Input: dimensioned drawing with shaded views. Units: mm. Origin: part minimum x, y, z. Give positions to 0.01 mm unless a question says otherwise; leave off trailing zeros. Order: outer loops, then holes, each group sorted by start corner. A loop starts at its lowest first (then second) coordinate and runs counter-clockwise, first axis right, second up. Notation, with made-up numbers: M -10.5,31.25 L 46.5,31.25 A15 cw 46.5,45.25 Z; hole C -3,82.25 d10. An arc over 180 degrees is marked long. Answer in a Markdown table with one row per item. Add a question column.
(1) Section query A-A, the plane y = 5. Return loops of the section in (x, z), plus the area to 3 significant figures.
(2) Section query C-C, the plane x = 18. Return loops of the section in (y, z), plus the area to 3 significant figures.
(3) Pin query (flat end, axial travel): P1, Ø2.5, axis at y = 5, z = 5, coming from the -X side. Return the tip coordinate at first contact, or that it passes through.
(4) Material intervals for line 1 along Y through (x, z) = (22.5, 5); line 2 along Y through (x, z) = (74.5, 6), sorted ascending.
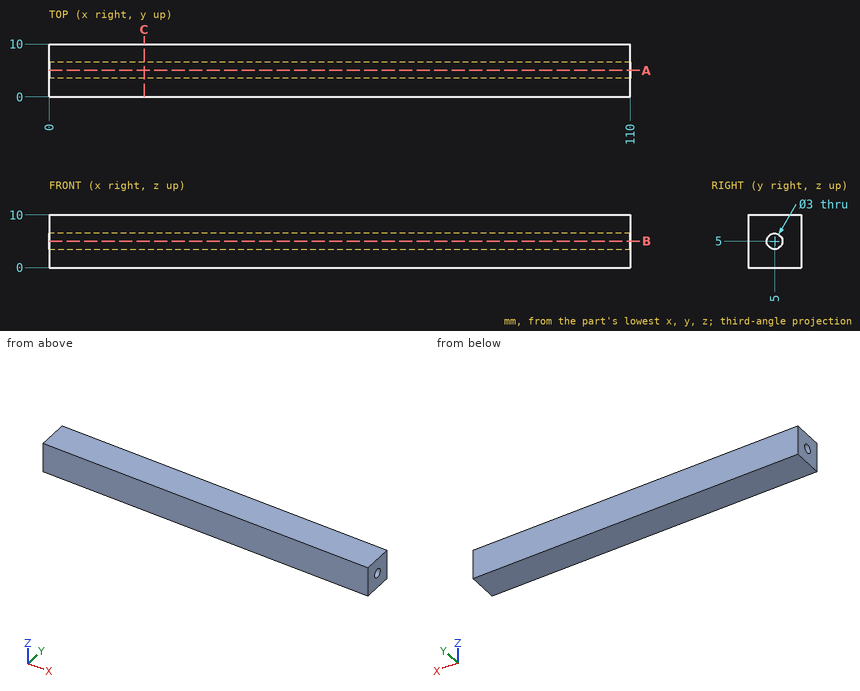
Values follow:
| question | item | result |
|---|---|---|
| 1 | outline | M 0,0 L 110,0 L 110,3.5 L 0,3.5 Z; M 0,6.5 L 110,6.5 L 110,10 L 0,10 Z |
| 1 | area | 770 mm² |
| 2 | outline | M 0,0 L 10,0 L 10,10 L 0,10 Z; hole C 5,5 d3 |
| 2 | area | 92.9 mm² |
| 3 | P1 | passes through |
| 4 | line 1 | y = 0 to 3.5, 6.5 to 10 |
| 4 | line 2 | y = 0 to 3.88, 6.12 to 10 |
